CAD build for the part. Positions are in the model's coordinates, mm. A direction names the side the tool comes from. Coordinates: 2 decimals unless noted, no trailing zeros. Order: outer loops, then holes, each group sorted by start corner. A loop starts at its lowest first (then second) coordinate and runs counter-clockwise, first axis right, second up. Notation, with made-up numbers: M 0,-24.75 L 46,-24.75 A19 cw 46,-0.75 Z; hole C 20,7 d9. An arc over 180 degrees is marked long. One line per item, written item: value.
from build123d import *

# Parameters (mm, degrees)
EXTRUDE_1_DEPTH             = 85
EXTRUDE_798_DEPTH           = 440
EXTRUDE_2_DEPTH             = 85
EXTRUDE_1413_DEPTH          = 85
EXTRUDE_1413_DEPTH_BACK     = 140
SKETCH_10_W                 = 210
SKETCH_10_H                 = 190
SKETCH_5_R                  = 115
CUT_EXTRUDE_1475_DEPTH      = 712.91642768
CUT_EXTRUDE_1609_REACH      = 710.683
CUT_EXTRUDE_1609_END_RADIUS = 115
SKETCH_12_R                 = 85
CUT_EXTRUDE_2000_REACH      = 739.219
SKETCH_13_R                 = 10
SKETCH_14_R                 = 5
CUT_EXTRUDE_6_DEPTH         = 30
FILLET_2_R                  = 10
FILLET_3_R                  = 10


with BuildPart() as part:
    # Эскиз2 → Боковой многогранник 1 (new body)
    with BuildSketch(Plane(origin=(0, 0, 0), x_dir=(1, 0, 0), z_dir=(0, 1, 0))):
        Polygon((0, 176.091832103), (-152.5, 88.045916051), (-152.5, -88.045916051), (0, -176.091832103), (152.5, -88.045916051), (152.5, 88.045916051), align=None)
    extrude(amount=EXTRUDE_1_DEPTH)

    # Sketch 344 → Extrude 798 (add)
    with BuildSketch(Plane(origin=(0, 0, 0), x_dir=(1, 0, 0), z_dir=(0, 1, 0))):
        Polygon((0, 161.658075373), (-140, 80.829037687), (-140, -80.829037687), (-47.5, -134.233937587), (-47.5, -195), (-132.5, -195), (-132.5, -290), (132.5, -290), (132.5, -195), (47.5, -195), (47.5, -134.233937587), (140, -80.829037687), (140, 80.829037687), align=None)
    extrude(amount=-EXTRUDE_798_DEPTH)

    # Эскиз4 → Боковой многогранник 2 (add)
    with BuildSketch(Plane.XZ.offset(440)):
        Polygon((0, -176.091832103), (152.5, -88.045916051), (152.5, 88.045916051), (0, 176.091832103), (-152.5, 88.045916051), (-152.5, -88.045916051), align=None)
    extrude(amount=EXTRUDE_2_DEPTH)

    # Эскиз10 → Extrude 1413 (add, two sides: drawn at the far end of the back side and taken through both)
    with BuildSketch(Plane(origin=(140, 0, 0), x_dir=(0, 0, -1), z_dir=(1, 0, 0)).offset(-EXTRUDE_1413_DEPTH_BACK)):
        with Locations((0, -305)):
            Rectangle(SKETCH_10_W, SKETCH_10_H)
    extrude(amount=EXTRUDE_1413_DEPTH + EXTRUDE_1413_DEPTH_BACK)

    # Эскиз5 → Cut-Extrude 1475 (cut, through all)
    with BuildSketch(Plane(origin=(0, 85, 0), x_dir=(1, 0, 0), z_dir=(0, 1, 0))):
        with Locations(Location((0, 0, 0), (0, 0, 270))):
            Circle(SKETCH_5_R)
    extrude(amount=-CUT_EXTRUDE_1475_DEPTH, mode=Mode.SUBTRACT)

    # Cut-Extrude 1609: up to this cylinder (the profile starts outside it)
    cut_extrude_1609_end = Plane(origin=(0, -305, 0), z_dir=(0, 1, 0)) * Cylinder(CUT_EXTRUDE_1609_END_RADIUS, 1652.366, mode=Mode.PRIVATE)
    # Эскиз12 → Cut-Extrude 1609 (cut, up to the surface)
    with BuildSketch(Plane(origin=(225, 0, 0), x_dir=(0, 0, -1), z_dir=(1, 0, 0)), mode=Mode.PRIVATE) as cut_extrude_1609_sk1:
        with Locations((0, -305)):
            Circle(SKETCH_12_R)
    cut_extrude_1609_tool1 = extrude(cut_extrude_1609_sk1.sketch, amount=-CUT_EXTRUDE_1609_REACH, mode=Mode.PRIVATE) - cut_extrude_1609_end
    add(cut_extrude_1609_tool1.solids().sort_by_distance((225, -305, 0))[0], mode=Mode.SUBTRACT)

    # Эскиз13 → Cut-Extrude 2000 (cut, up to next)
    with BuildSketch(Plane.XY.offset(290), mode=Mode.PRIVATE) as cut_extrude_2000_sk1:
        with Locations((-112.5, -420)):
            Circle(SKETCH_13_R)
    cut_extrude_2000_tool1 = extrude(cut_extrude_2000_sk1.sketch, amount=-CUT_EXTRUDE_2000_REACH, mode=Mode.PRIVATE) & part.part
    # Эскиз13 → Cut-Extrude 2000 (cut, up to next)
    with BuildSketch(Plane.XY.offset(290), mode=Mode.PRIVATE) as cut_extrude_2000_sk2:
        with Locations((112.5, -420)):
            Circle(SKETCH_13_R)
    cut_extrude_2000_tool2 = extrude(cut_extrude_2000_sk2.sketch, amount=-CUT_EXTRUDE_2000_REACH, mode=Mode.PRIVATE) & part.part
    # Эскиз13 → Cut-Extrude 2000 (cut, up to next)
    with BuildSketch(Plane.XY.offset(290), mode=Mode.PRIVATE) as cut_extrude_2000_sk3:
        with Locations((-112.5, -20)):
            Circle(SKETCH_13_R)
    cut_extrude_2000_tool3 = extrude(cut_extrude_2000_sk3.sketch, amount=-CUT_EXTRUDE_2000_REACH, mode=Mode.PRIVATE) & part.part
    # Эскиз13 → Cut-Extrude 2000 (cut, up to next)
    with BuildSketch(Plane.XY.offset(290), mode=Mode.PRIVATE) as cut_extrude_2000_sk4:
        with Locations((112.5, -20)):
            Circle(SKETCH_13_R)
    cut_extrude_2000_tool4 = extrude(cut_extrude_2000_sk4.sketch, amount=-CUT_EXTRUDE_2000_REACH, mode=Mode.PRIVATE) & part.part
    add(cut_extrude_2000_tool1.solids().sort_by_distance((-112.5, -420, 290))[0], mode=Mode.SUBTRACT)
    add(cut_extrude_2000_tool2.solids().sort_by_distance((112.5, -420, 290))[0], mode=Mode.SUBTRACT)
    add(cut_extrude_2000_tool3.solids().sort_by_distance((-112.5, -20, 290))[0], mode=Mode.SUBTRACT)
    add(cut_extrude_2000_tool4.solids().sort_by_distance((112.5, -20, 290))[0], mode=Mode.SUBTRACT)

    # Эскиз14 → Вырез-Вытянуть6 (cut)
    with BuildSketch(Plane(origin=(225, 0, 0), x_dir=(0, 0, -1), z_dir=(1, 0, 0))):
        with Locations((95, -220)):
            Circle(SKETCH_14_R)
        with Locations((95, -390)):
            Circle(SKETCH_14_R)
        with Locations((-95, -220)):
            Circle(SKETCH_14_R)
        with Locations((-95, -390)):
            Circle(SKETCH_14_R)
    extrude(amount=-CUT_EXTRUDE_6_DEPTH, mode=Mode.SUBTRACT)

    # Скругление2
    fillet_2_edges = [part.edges().sort_by_distance(p)[0] for p in [
        (132.5, -440, 242.5),
        (-132.5, -440, 242.5),
        (-132.5, 0, 242.5),
        (132.5, 0, 242.5),
    ]]
    fillet(fillet_2_edges, radius=FILLET_2_R)

    # Скругление3
    fillet_3_edges = [part.edges().sort_by_distance(p)[0] for p in [
        (161.567332603, -210, -105),
        (161.567332603, -400, -105),
        (161.567332603, -400, 105),
        (161.567332603, -210, 105),
    ]]
    fillet(fillet_3_edges, radius=FILLET_3_R)


solid = part.part
Q1. Slice it at D-D (y = -108.5). List the corners of the cut face in (x, z).
Recorded:
outline: M -140,-80.83 L 0,-161.66 L 140,-80.83 L 140,80.83 L 47.5,134.23 L 47.5,195 L 132.5,195 L 132.5,290 L -132.5,290 L -132.5,195 L -47.5,195 L -47.5,134.23 L -140,80.83 Z; hole C 0,0 d230
Q2. Slice it at A-A (z = 0). List the corners of the cut face in (x, y), plus the area to 3 significant figures.
Recorded:
outline: M -152.5,-525 L -115,-525 L -115,85 L -152.5,85 L -152.5,0 L -140,0 L -140,-440 L -152.5,-440 Z; M 115,-525 L 152.5,-525 L 152.5,-440 L 140,-440 L 140,-400 L 225,-400 L 225,-390 L 115,-390 Z; M 115,-220 L 225,-220 L 225,-210 L 140,-210 L 140,0 L 152.5,0 L 152.5,85 L 115,85 Z
area: 32,200 mm^2
Q3. Pin check, flat tips, straight feed: pin 1 Ø12 at (y, z) = (-164.5, 185) entering from +X; pin 2 Ø3 at (y, z) = (-221.5, 95) entering from +X; pin 3 Ø3 at (y, z) = (-25, 17.5) entering from -X. Stop position of each tip, or through.
Recorded:
pin 1: stops at x = 47.5
pin 2: stops at x = 195
pin 3: stops at x = -140
Q4. Drill centre lines: line 1 along Y through (x, z) = (211, 95); line 2 along Y through (x, z) = (-112, 254); line 3 along Z through (x, y) = (-70, -274). Where is each one in solid material? Low to high.
Recorded:
line 1: y = -400 to -395, -385 to -225, -215 to -210
line 2: y = -440 to -429.99, -410.01 to -29.99, -10.01 to 0
line 3: z = -121.24 to -91.24, 91.24 to 121.24, 195 to 290
Q5. Mould opens along X. For faces 1 (the face through (-102.4, 85, -53)), 2 (the face through (-113.802, -410.085, 243.165)), 3 (the face through (152.5, -482, -1)) say: released by +X, released by -X, zero draft, split by the parting line, or undercut.
Recorded:
face 1: zero draft
face 2: undercut
face 3: released by +X
Q6. Which spindle directions (+Z, -Z, +X, -X, +Y, -Y) get a long thin tool onto all of the face, cutting with end or side? Do faces 4 (the face through (168.7, -337.6, -78.5)), 5 (the face through (-57, -440, -133)), 6 (the face through (161, -306, -105)). Say none if no direction does.
Recorded:
face 4: +X
face 5: none
face 6: -Z, +X
Q7. Slice it at B-B (z = 218). List the corners of the cut face in (x, y), plus the area to 3 significant figures.
Recorded:
outline: M -132.5,-430 A10 ccw -122.5,-440 L 122.5,-440 A10 ccw 132.5,-430 L 132.5,-10 A10 ccw 122.5,0 L -122.5,0 A10 ccw -132.5,-10 Z; hole C -112.5,-420 d20; hole C -112.5,-20 d20; hole C 112.5,-420 d20; hole C 112.5,-20 d20
area: 115,000 mm^2
Q8. Slice it at C-C (x = 187.5). List the corners of the cut face in (y, z).
Recorded:
outline: M -400,-95 A10 ccw -390,-105 L -220,-105 A10 ccw -210,-95 L -210,95 A10 ccw -220,105 L -390,105 A10 ccw -400,95 Z; hole C -305,0 d170
